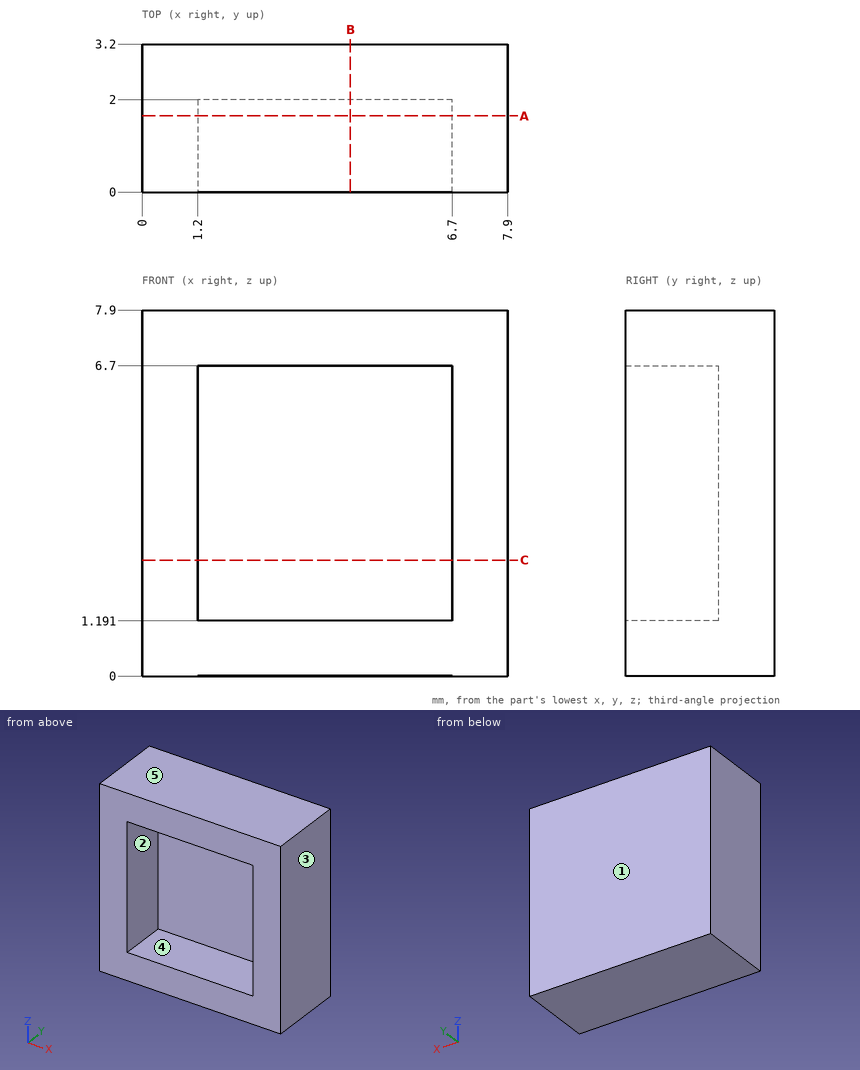
Here's the drawing with two shaded views (mm, measured from the low corner). I have some questions. A direction names the side the tool comes from. Give positions to 0.01 mm unless a question says otherwise; leave off trailing zeros. Order: outer loops, then holes, each group sorted by start corner. A loop starts at its lowest first (then second) coordinate and runs counter-clockwise, first axis right, second up. Notation, with made-up numbers: (61, -35.5) -> (104, -35.5) arc R26 ccw to (104, -14.5) -> close; hole circle Ø6 at (-1, 24). An arc over 180 degrees is marked (long way). Use a Markdown table: item, result. Add a question column.
Item 1: For the marked faces 1 and 2, which set-ups out of +Z, -Z, +X, -X, +Y, -Y let a thin tool reach every point of the face, with its end or its side?
Item 2: Imagine slicing it at C-C on z = 2.5. Please give me the cut outline in (x, y), plus the area to 3 significant figures.
Item 3: I need wall thicknesses on line 1 (Z direction, x = 1.75, y = 1.4); line 2 (X direction, y = 1.55, z = 3.75); line 3 (Y direction, x = 5, z = 6). Which ranges of each line are inside material? Lowest first, please.
Item 4: If we mould it in two halves opening along Z, with no side actions, what happens to the marked faces 3, 4 and 5? For each: pulls with the +Z half, pulls with the -Z half, needs draft (parallel to the pull), parting line crosses it, or undercut.
Item 5: Imagine slicing it at B-B on x = 4.5. Please give me the cut outline in (y, z), plus the area to 3 significant figures.
Item 6: Will this pin go through, and if not, where does the flat tip stop? pin 1 (4.5 mm diameter, centred on x = 4, z = 3, fed in from -Y).
Item 7: Imagine slicing it at A-A on y = 1.65. Please give me the cut outline in (x, z), plus the area to 3 significant figures.
Data:
| question | item | result |
|---|---|---|
| 1 | face 1 | +Z, -Z, +X, -X, +Y |
| 1 | face 2 | -Y |
| 2 | outline | (0, 0) -> (1.2, 0) -> (1.2, 2) -> (6.7, 2) -> (6.7, 0) -> (7.9, 0) -> (7.9, 3.2) -> (0, 3.2) -> close |
| 2 | area | 14.3 mm² |
| 3 | line 1 | z = 0 to 1.19, 6.7 to 7.9 |
| 3 | line 2 | x = 0 to 1.2, 6.7 to 7.9 |
| 3 | line 3 | y = 2 to 3.2 |
| 4 | face 3 | needs draft |
| 4 | face 4 | undercut |
| 4 | face 5 | pulls with the +Z half |
| 5 | outline | (0, 0) -> (3.2, 0) -> (3.2, 7.9) -> (0, 7.9) -> (0, 6.7) -> (2, 6.7) -> (2, 1.19) -> (0, 1.19) -> close |
| 5 | area | 14.3 mm² |
| 6 | pin 1 | stops at y = 0 |
| 7 | outline | (0, 0) -> (7.9, 0) -> (7.9, 7.9) -> (0, 7.9) -> close; hole (1.2, 1.19) -> (6.7, 1.19) -> (6.7, 6.7) -> (1.2, 6.7) -> close |
| 7 | area | 32.1 mm² |
